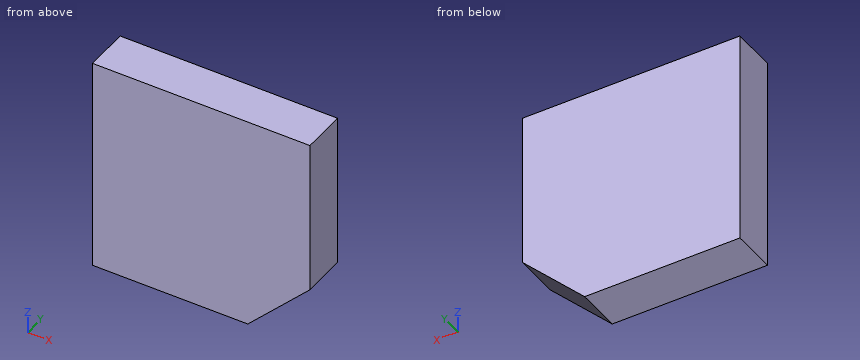
from build123d import *

# Parameters (mm, degrees)
SKETCH1_W           = 88.9
SKETCH1_H           = 88.9
BOSS_EXTRUDE1_DEPTH = 18.25625
CUT_EXTRUDE1_DEPTH  = 66.459114446


with BuildPart() as part:
    # Sketch1 → Boss-Extrude1 (new body)
    with BuildSketch(Plane(origin=(0, 0, 0), x_dir=(1, 0, 0), z_dir=(0, 1, 0))):
        Rectangle(SKETCH1_W, SKETCH1_H)
    extrude(amount=BOSS_EXTRUDE1_DEPTH)

    # Sketch2 → Cut-Extrude1 (cut, through all)
    with BuildSketch(Plane(origin=(0, 18.25625, 0), x_dir=(1, 0, 0), z_dir=(0, 1, 0))):
        Polygon((44.45, 44.45), (44.45, 19.05), (19.05, 44.45), align=None)
    extrude(amount=-CUT_EXTRUDE1_DEPTH, mode=Mode.SUBTRACT)


solid = part.part
Geometry: final body of the model. Coordinates: model frame, mm. Give positions to 0.01 mm unless a question says otherwise; leave off trailing zeros. Order: outer loops, then holes, each group sorted by start corner. A loop starts at its lowest first (then second) coordinate and runs counter-clockwise, first axis right, second up. Notation, with made-up numbers: (69.5, -28.75) -> (101.5, -28.75) arc R21 cw to (101.5, -10.75) -> close; hole circle Ø6 at (38, 6.25). An arc over 180 degrees is marked (long way). Answer as a JSON object with one key per item and string values.
Q1. Material intervals for probe 1 along Z at (x, y) = (36.5, 7); probe 2 along X at (y, z) = (14.25, -25); probe 3 along Z at (x, y) = (29, 15), sorted ascending.
Entries:
{"probe 1": "z = -27 to 44.45", "probe 2": "x = -44.45 to 38.5", "probe 3": "z = -34.5 to 44.45"}
Q2. Section C-C (x = 29.5). Output: boundary loops of the cut face in (y, z).
Entries:
{"outline": "(0, -34) -> (18.26, -34) -> (18.26, 44.45) -> (0, 44.45) -> close"}
Q3. Section A-A (y = 5). Output: boundary loops of the cut face in (x, z).
Entries:
{"outline": "(-44.45, -44.45) -> (19.05, -44.45) -> (44.45, -19.05) -> (44.45, 44.45) -> (-44.45, 44.45) -> close"}
Q4. Section B-B (z = -25.5). Output: boundary loops of the cut face in (x, y).
Entries:
{"outline": "(-44.45, 0) -> (38, 0) -> (38, 18.26) -> (-44.45, 18.26) -> close"}
